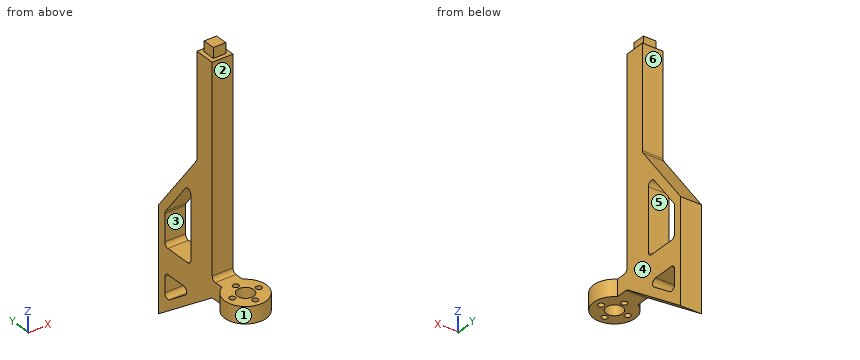
```python
from build123d import *

# Parameters (mm, degrees)
SKETCH1_R           = 5.08
SKETCH1_R_2         = 1.778
BOSS_EXTRUDE1_DEPTH = 10.16
SKETCH3_W           = 12.7
SKETCH3_H           = 12.7
BOSS_EXTRUDE2_DEPTH = 127
SKETCH6_W           = 7.62
SKETCH6_H           = 7.62
BOSS_EXTRUDE3_DEPTH = 6.35
BOSS_EXTRUDE4_START = -12.7
BOSS_EXTRUDE4_DEPTH = 12.7
FILLET2_R           = 2.54
BOSS_EXTRUDE5_START = -12.7
BOSS_EXTRUDE5_DEPTH = 12.7
FILLET3_R           = 2.54


with BuildPart() as part:
    # Sketch1 → Boss-Extrude1 (new body)
    with BuildSketch(Plane.XY):
        with BuildLine():
            Line((-6.35, 12.7), (-6.35, 10.998522628))
            ThreePointArc((-6.35, 10.998522628), (0, -12.7), (6.35, 10.998522628))
            Line((6.35, 10.998522628), (6.35, 12.7))
            Line((6.35, 12.7), (6.35, 63.5))
            Line((6.35, 63.5), (-6.35, 63.5))
            Line((-6.35, 63.5), (-6.35, 12.7))
        make_face()
        Circle(SKETCH1_R, mode=Mode.SUBTRACT)
        with Locations((0, 8.128)):
            Circle(SKETCH1_R_2, mode=Mode.SUBTRACT)
        with Locations((8.128, 0)):
            Circle(SKETCH1_R_2, mode=Mode.SUBTRACT)
        with Locations((0, -8.128)):
            Circle(SKETCH1_R_2, mode=Mode.SUBTRACT)
        with Locations((-8.128, 0)):
            Circle(SKETCH1_R_2, mode=Mode.SUBTRACT)
    extrude(amount=BOSS_EXTRUDE1_DEPTH)

    # Sketch3 → Boss-Extrude2 (add)
    with BuildSketch(Plane.XY.offset(10.16)):
        with Locations((0, 25.4)):
            Rectangle(SKETCH3_W, SKETCH3_H)
    extrude(amount=BOSS_EXTRUDE2_DEPTH)

    # Sketch6 → Boss-Extrude3 (add)
    with BuildSketch(Plane.XY.offset(137.16)):
        with Locations((0, 25.4)):
            Rectangle(SKETCH6_W, SKETCH6_H)
    extrude(amount=BOSS_EXTRUDE3_DEPTH)

    # Sketch5 → Boss-Extrude4 (add)
    with BuildSketch(Plane.ZY.offset(6.35).offset(BOSS_EXTRUDE4_START)):
        Polygon((10.16, 63.5), (31.75, 63.5), (73.66, 31.75), (10.16, 31.75), (10.16, 36.83), (58.541821836, 36.83), (30.043021836, 58.42), (10.16, 58.42), align=None)
    extrude(amount=BOSS_EXTRUDE4_DEPTH)

    # Fillet2
    fillet2_edges = [part.edges().sort_by_distance(p)[0] for p in [
        (0, 31.75, 73.66),
    ]]
    fillet(fillet2_edges, radius=FILLET2_R)

    # Sketch7 → Boss-Extrude5 (add)
    with BuildSketch(Plane(origin=(6.35, 0, 0), x_dir=(0, 0, -1), z_dir=(1, 0, 0)).offset(BOSS_EXTRUDE5_START)):
        Polygon((0, 63.5), (0, 19.05), (31.75, 63.5), align=None)
        Polygon((5.08, 58.42), (21.878598235, 58.42), (5.08, 34.901962471), align=None, mode=Mode.SUBTRACT)
    extrude(amount=BOSS_EXTRUDE5_DEPTH)

    # Fillet3
    fillet3_edges = [part.edges().sort_by_distance(p)[0] for p in [
        (0, 19.05, 0),
        (0, 34.901962471, -5.08),
        (0, 58.42, -5.08),
        (0, 58.42, -21.878598235),
        (0, 19.05, 10.16),
        (0, 58.42, 10.16),
        (0, 58.42, 30.043021836),
        (0, 36.83, 58.541821836),
        (0, 36.83, 10.16),
    ]]
    fillet(fillet3_edges, radius=FILLET3_R)


solid = part.part
```
Can you work these out from the model? Positions are in its coordinate system, mm. Face numbers are marked on the shaded views. A direction names the side the tool comes from. Round coordinates to 2 decimals unless told otherwise and drop trailing zeros. Order: outer loops, then holes, each group sorted by start corner. A loop starts at its lowest first (then second) coordinate and runs counter-clockwise, first axis right, second up. Notation, with made-up numbers: (-11.5, 36.25) -> (20.5, 36.25) arc R8 ccw to (20.5, 48.25) -> close; hole circle Ø9 at (49, 4.25). An arc over 180 degrees is marked (long way). Return JSON: item names as keys, results as strings. Group by question number.
1. If we section it at A-A, the plane y = 0: Write out the boundary of the cut face in (x, z), then the cut area to 3 significant figures.
2. Which directions (+Z, -Z, +X, -X, +Y, -Y) give clear straight access to the entire face, cutting with the end or side of a thin tool? Please do the marked faces 1, 2 and 3.
3. If we section it at C-C, the plane x = 0: Count the separate pieces of the cut face and the enclosed holes in it, then the cut area to 3 significant figures.
4. Will these pins go through, and if not, where does the flat tip stop? pin 1 (3 mm diameter, centred on x = -1.5, z = 140.5, fed in from -Y); pin 2 (4 mm diameter, centred on x = -2.5, z = 119, fed in from +Y); pin 3 (5.5 mm diameter, centred on x = 0, y = -8.128, fed in from -Z); pin 4 (3 mm diameter, centred on x = -8.128, y = 0, fed in from +Z).
5. We'd pull the mould along Y, two halves only. Please class the marked faces 4, 5 and 6: released by +Y, released by -Y, zero draft, split by the parting line, or undercut.
6. If we section it at D-D, the plane y = 45.5: Write out the boundary of the cut face in (x, z), then the cut area to 3 significant figures.
7. I need wall thicknesses on line 1 (Y direction, x = 0, z = 2); line 2 (Z direction, x = 3.75, y = 11.5); line 3 (Y direction, x = 4.75, z = 12.5). Which ranges of each line are inside material? Lowest first, please. Write a range as [from, to].
8. If we section it at B-B, the plane z = 21: Write out the boundary of the cut face in (x, y).
Output values:
{
 "1": {"outline": "(-12.7, 0) -> (-9.91, 0) -> (-9.91, 10.16) -> (-12.7, 10.16) -> close; (-6.35, 0) -> (-5.08, 0) -> (-5.08, 10.16) -> (-6.35, 10.16) -> close; (5.08, 0) -> (6.35, 0) -> (6.35, 10.16) -> (5.08, 10.16) -> close; (9.91, 0) -> (12.7, 0) -> (12.7, 10.16) -> (9.91, 10.16) -> close", "area": "82.6 mm²"},
 "2": {"face 1": "+Z, -Z", "face 2": "+Z, +X, -X, -Y", "face 3": "+X, -X"},
 "3": {"separate pieces": "4", "enclosed holes": "2", "area": "3,420 mm²"},
 "4": {"pin 1": "y = 21.59", "pin 2": "y = 31.75", "pin 3": "z = 0", "pin 4": "through"},
 "5": {"face 4": "zero draft", "face 5": "undercut", "face 6": "released by +Y"},
 "6": {"outline": "(-6.35, -18.89) -> (6.35, -18.89) -> (6.35, -12.65) -> (-6.35, -12.65) -> close; (-6.35, -5.08) -> (6.35, -5.08) -> (6.35, 10.16) -> (-6.35, 10.16) -> close; (-6.35, 47.1) -> (6.35, 47.1) -> (6.35, 55.51) -> (-6.35, 55.51) -> close", "area": "380 mm²"},
 "7": {"line 1": "[-12.7, -9.91], [-6.35, -5.08], [5.08, 6.35], [9.91, 63.5]", "line 2": "[0, 10.16]", "line 3": "[19.04, 36.84], [58.41, 63.5]"},
 "8": {"outline": "(-6.35, 19.05) -> (6.35, 19.05) -> (6.35, 36.83) -> (-6.35, 36.83) -> close; (-6.35, 58.42) -> (6.35, 58.42) -> (6.35, 63.5) -> (-6.35, 63.5) -> close"}
}
